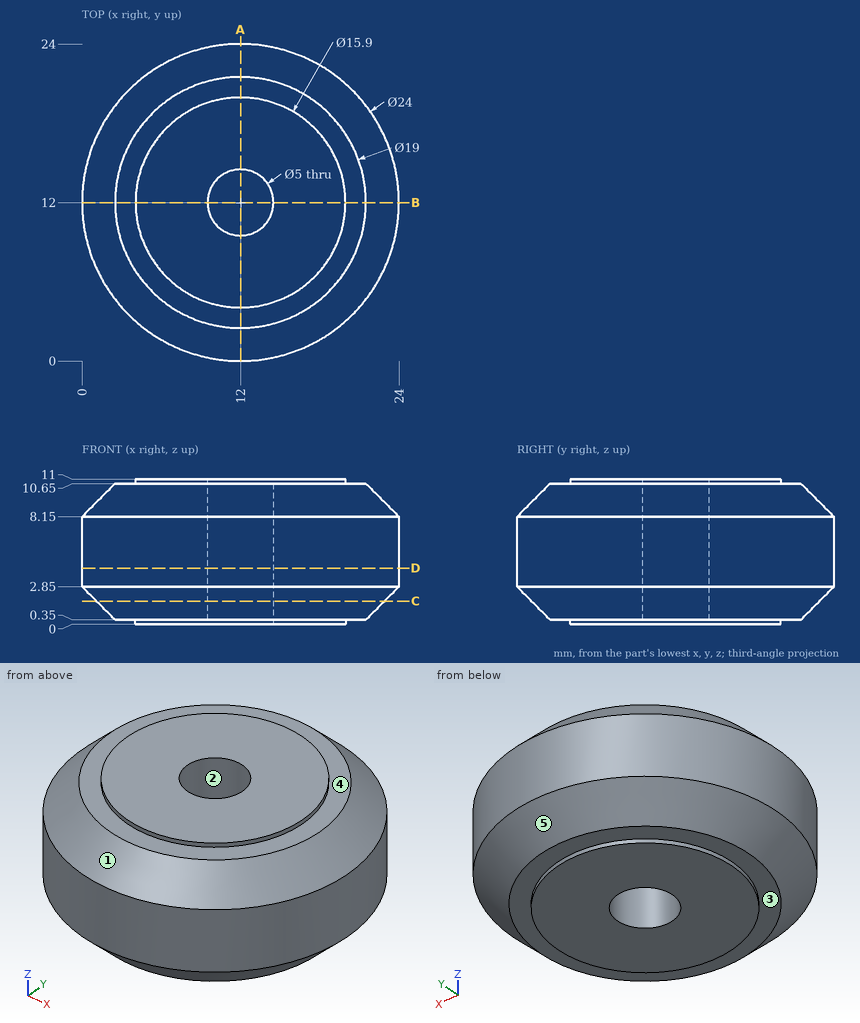
Here's the drawing with two shaded views (mm, measured from the low corner). I have some questions. A direction names the side the tool comes from. Give positions to 0.01 mm unless a question says otherwise; leave off trailing zeros. Loops run counter-clockwise (first coordinate to the right, second up) from the corner with the lowest first, then second, coordinate; pieces in that order, holes last. Notation, with made-up numbers: (49, 30) -> (54, 30) arc R17 ccw to (54, 49) -> close; hole circle Ø5 at (60.25, 2). An arc over 180 degrees is marked (long way). Answer as a JSON object with one key per item and string values. Group by question number.
Item 1: Imagine slicing it at C-C on z = 1.75. Write out the boundary of the cut face in (x, y).
Item 2: Imagine slicing it at D-D on z = 4.25. Write out the boundary of the cut face in (x, y).
Item 3: I need wall thicknesses on L1, parallel to Y at x = 12, z = 4.75; L2, parallel to X at y = 14, z = 4.25; L3, parallel to X at y = 1.5, z = 8. Which ranges of each line are inside material? Lowest first, please.
Item 4: Thinking about a two-plate mould opening in X: for the marked faces 1, 2 and 3, which applies, pulls with the +X half, pulls with the -X half, needs draft (parallel to the pull), parting line crosses it, or undercut?
Item 5: On a 3-axis mill with a long thin cutter (end or side, diameter ignored), from which of +Z, -Z, +X, -X, +Y, -Y can I reach the whole of each face in a straight line? I mean the marked faces 4 and 5. Say none if no direction works.
Item 6: Imagine slicing it at A-A on x = 12. Write out the boundary of the cut face in (y, z), then the cut area to 3 significant figures.
Item 7: Will these pins go through, and if not, where does the flat tip stop? pin 1 (1.5 mm diameter, centred on y = 18, z = 6.5, fed in from -X); pin 2 (2 mm diameter, centred on y = 9, z = 4, fed in from +X); pin 3 (6 mm diameter, centred on x = 15.5, z = 3.5, fed in from -Y).
Answer list:
{
 "1": {"outline": "circle Ø21.8 at (12, 12); hole circle Ø5 at (12, 12)"},
 "2": {"outline": "circle Ø24 at (12, 12); hole circle Ø5 at (12, 12)"},
 "3": {"L1": "y = 0 to 9.5, 14.5 to 24", "L2": "x = 0.17 to 10.5, 13.5 to 23.83", "L3": "x = 6.19 to 17.81"},
 "4": {"face 1": "parting line crosses it", "face 2": "undercut", "face 3": "needs draft"},
 "5": {"face 4": "+Z", "face 5": "-Z"},
 "6": {"outline": "(0, 2.85) -> (2.5, 0.35) -> (4.05, 0.35) -> (4.05, 0) -> (9.5, 0) -> (9.5, 11) -> (4.05, 11) -> (4.05, 10.65) -> (2.5, 10.65) -> (0, 8.15) -> close; (14.5, 0) -> (19.95, 0) -> (19.95, 0.35) -> (21.5, 0.35) -> (24, 2.85) -> (24, 8.15) -> (21.5, 10.65) -> (19.95, 10.65) -> (19.95, 11) -> (14.5, 11) -> close", "area": "191 mm2"},
 "7": {"pin 1": "stops at x = 1.21", "pin 2": "stops at x = 23.83", "pin 3": "stops at y = 0.01"}
}
